Source: CAD feature listing. Evaluate the final solid. Frame: model axes, mm. A direction names the side the tool comes from. Round coordinates to 2 decimals unless told otherwise and drop trailing zeros. Write each loop counter-clockwise with the first axis right and the second up, starting at its lowest first coordinate (ties: lowest second). Pieces come first, ordered by that corner, then holes. Notation, with made-up numbers: (64, 34.25) -> (102, 34.25) arc R34 cw to (102, 72.25) -> close; hole circle Ø6 at (8, 60). An arc over 180 degrees is marked (long way). Put each result on its own line as item: value.
```python
from build123d import *

# Parameters (mm, degrees)
SKETCH1_R           = 75
BOSS_EXTRUDE1_DEPTH = 3
SKETCH2_R           = 1.75
CUT_EXTRUDE1_DEPTH  = 107.108435103
SKETCH3_R           = 40.5
SKETCH3_R_2         = 37.5
BOSS_EXTRUDE2_DEPTH = 3
SKETCH4_W           = 3
SKETCH4_H           = 30
CUT_EXTRUDE2_DEPTH  = 107.235587258


with BuildPart() as part:
    # Sketch1 → Boss-Extrude1 (new body)
    with BuildSketch(Plane.XY):
        Circle(SKETCH1_R)
    extrude(amount=BOSS_EXTRUDE1_DEPTH)

    # Sketch2 → Cut-Extrude1 (cut, through all)
    with BuildSketch(Plane.XY.offset(3)):
        with Locations((-50, 15)):
            Circle(SKETCH2_R)
        with Locations((-50, -15)):
            Circle(SKETCH2_R)
        with Locations((50, -15)):
            Circle(SKETCH2_R)
        with Locations((50, 15)):
            Circle(SKETCH2_R)
        Circle(SKETCH2_R)
    extrude(amount=-CUT_EXTRUDE1_DEPTH, mode=Mode.SUBTRACT)

    # Sketch3 → Boss-Extrude2 (add)
    with BuildSketch(Plane.XY.offset(3)):
        Circle(SKETCH3_R)
        Circle(SKETCH3_R_2, mode=Mode.SUBTRACT)
    extrude(amount=BOSS_EXTRUDE2_DEPTH)

    # Sketch4 → Cut-Extrude2 (cut, through all)
    with BuildSketch(Plane(origin=(0, 0, 0), x_dir=(-1, 0, 0), z_dir=(0, 0, -1))):
        with Locations((-26.5, -50)):
            Rectangle(SKETCH4_W, SKETCH4_H)
        with Locations((26.5, -50)):
            Rectangle(SKETCH4_W, SKETCH4_H)
    extrude(amount=-CUT_EXTRUDE2_DEPTH, mode=Mode.SUBTRACT)


solid = part.part
```
Q1. Pin query (flat end, axial travel): pin 1 (0.9 mm diameter, centred on y = -55, z = 2, fed in from -X); pin 2 (1.5 mm diameter, centred on x = -27, z = 1.5, fed in from +Y); pin 3 (0.9 mm diameter, centred on x = 27, z = 1, fed in from +Y). Return the tip coordinate at first contact, or that it passes through.
Ans:
pin 1: stops at x = -51.47
pin 2: stops at y = 70.26
pin 3: stops at y = 70.14
Q2. Material intervals for line 1 (Y direction, x = 50.5, z = 2.95); line 2 (Y direction, x = -50, z = 1.85); line 3 (Z direction, x = -51, y = -8), sorted ascending. Write a range as [from, to].
Ans:
line 1: y = [-55.45, -16.68], [-13.32, 13.32], [16.68, 55.45]
line 2: y = [-55.9, -16.75], [-13.25, 13.25], [16.75, 55.9]
line 3: z = [0, 3]
Q3. Cut plane C-C on z = 4.8. Output: boundary loops of the cut face in (x, y), and give its area (3 significant figures).
Ans:
outline: circle Ø81 at (0, 0); hole circle Ø75 at (0, 0)
area: 735 mm^2
Q4. Reachability of faces 1 (the cylindrical face through (-4.88, 37.18, 4.48)), 2 (the cylindrical face through (51.669, 15.526, 1.521)) from +Z, -Z, +X, -X, +Y, -Y: full face, straight path, thin tool, end or side. Return the list, or none.
Ans:
face 1: +Z
face 2: +Z, -Z
Q5. Cut plane D-D on y = -15. Output: boundary loops of the cut face in (x, z), and give its area (3 significant figures).
Ans:
outline: (-73.48, 0) -> (-51.75, 0) -> (-51.75, 3) -> (-73.48, 3) -> close; (-48.25, 0) -> (48.25, 0) -> (48.25, 3) -> (37.62, 3) -> (37.62, 6) -> (34.37, 6) -> (34.37, 3) -> (-34.37, 3) -> (-34.37, 6) -> (-37.62, 6) -> (-37.62, 3) -> (-48.25, 3) -> close; (51.75, 0) -> (73.48, 0) -> (73.48, 3) -> (51.75, 3) -> close
area: 439 mm^2
Q6. Cut plane A-A on x = 0. Output: boundary loops of the cut face in (y, z).
Ans:
outline: (-75, 0) -> (-1.75, 0) -> (-1.75, 3) -> (-37.5, 3) -> (-37.5, 6) -> (-40.5, 6) -> (-40.5, 3) -> (-75, 3) -> close; (1.75, 0) -> (75, 0) -> (75, 3) -> (40.5, 3) -> (40.5, 6) -> (37.5, 6) -> (37.5, 3) -> (1.75, 3) -> close
Q7. Draft query along X for faces 3 (the flat face through (16, 1, 0)), 4 (the cylindrical face through (-9.764, 74.362, 1.479)), 5 (the cylindrical face through (-48.331, 15.526, 1.521)), 6 (the cylindrical face through (51.669, -14.474, 1.521)). Return one class per face: +X half, -X half, draft (parallel to the pull), parting line (faces both ways), or undercut.
Ans:
face 3: draft
face 4: parting line
face 5: undercut
face 6: undercut
